Work out the finished part from the listing and answer in its coordinate system (mm). Face numbers are marked on the shaded views. Coordinates: 2 decimals unless noted, no trailing zeros. Loops run counter-clockwise (first coordinate to the right, second up) from the corner with the lowest first, then second, coordinate; pieces in that order, holes last.
Autodesk Inventor part; units mm, degrees
ref_plane "YZ Plane" through (0, 0, 0) normal (1, 0, 0) x (0, 1, 0)
ref_plane "XZ Plane" through (0, 0, 0) normal (0, 1, 0) x (-1, 0, 0)
ref_plane "XY Plane" through (0, 0, 0) normal (0, 0, 1) x (1, 0, 0)
sketch "Sketch1" plane through (0, 0, 0) normal (0, 1, 0) x (-1, 0, 0)
  circle A0 centre (0, 0) radius 18.5
  dimension "d0" = 37
extrude "Extrusion1" add sketch "Sketch1" along normal blind 55.8
sketch "Sketch2" plane through (0, 55.8, 0) normal (0, 1, 0) x (1, 0, 0)
  circle A0 centre (0, 0) radius 6
  dimension "d3" = 12
extrude "Extrusion2" add sketch "Sketch2" along normal blind 5
sketch "Sketch3" plane through (0, 60.8, 0) normal (0, 1, 0) x (1, 0, 0)
  circle A0 centre (0, 0) radius 3
  line L0 (-2.5, -3) -> (3, -3)
  line L1 (3, -3) -> (3, 3)
  line L2 (3, 3) -> (-2.5, 3)
  line L3 (-2.5, 3) -> (-2.5, -3)
  point P0 (-2.5, 1.6583)
  point P1 (-2.5, -1.6583)
  dimension "d6" = 6
  dimension "d7" = 5.5
extrude "Extrusion3" add sketch "Sketch3" along normal blind 14 contours A0 L3 picked at (0.6006, -0.3482)
sketch "Sketch4" plane through (0, 0, 0) normal (0, -1, 0) x (1, 0, 0)
  circle A0 centre (0, 0) radius 17.5
  circle A1 centre (0, 0) radius 18.5
  dimension "d27" = 1
extrude "Extrusion4" cut sketch "Sketch4" against normal blind 1 contours A0
sketch "Sketch5" plane through (0, 1, 0) normal (0, -1, 0) x (1, 0, 0)
  circle A0 centre (0, 0) radius 18.5
  circle A1 centre (0, 0) radius 5
  dimension "d13" = 10
extrude "Extrusion5" add sketch "Sketch5" along normal blind 2 contours A1
sketch "Sketch7" plane through (0, 55.8, 0) normal (0, 1, 0) x (1, 0, 0)
  line L0 (0, 25.9) -> (0, -25.9)
  point P0 (0, 0)
  point P1 (0, 15.5)
  point P2 (-13.4234, 7.75)
  point P3 (-13.4234, -7.75)
  point P4 (0, -15.5)
  point P5 (13.4234, -7.75)
  point P6 (13.4234, 7.75)
  dimension "d35" = 15.5
  dimension "d38" = 360
hole "Hole1" at (-13.4234, 55.8, -7.75) at (-13.4234, 55.8, 7.75) at (13.4234, 55.8, 7.75) at (13.4234, 55.8, -7.75) at (0, 55.8, -15.5) at (0, 55.8, 15.5) direction (0, -1, 0) diameter 2.459 depth 8.8 tip angle 118
sketch "Sketch8" plane through (0, 1, 0) normal (0, -1, 0) x (1, 0, 0)
  line L0 (-11.5, -1.5) -> (-11, -1.5)
  line L1 (-11, -1.5) -> (-11, 1.5)
  line L2 (-11, 1.5) -> (-11.5, 1.5)
  line L3 (-11.5, 1.5) -> (-11.5, -1.5)
  line L4 (11, -1.5) -> (11.5, -1.5)
  line L5 (11.5, -1.5) -> (11.5, 1.5)
  line L6 (11.5, 1.5) -> (11, 1.5)
  line L7 (11, 1.5) -> (11, -1.5)
  circle A0 centre (0, 0) radius 5
  circle A1 centre (0, 0) radius 17.5
  line L8 (0, -17.5) -> (0, 17.5) construction
  point P0 (-11, 0)
  point P1 (11, 0)
  dimension "d30" = 23
  dimension "d31" = 0.5
  dimension "d32" = 0.5
  dimension "d33" = 3
  dimension "d34" = 3
extrude "Extrusion7" add sketch "Sketch8" along normal blind 6.5 contours L3 L2 L1 L0 | L7 L6 L5 L4
properties part number "Motor24V_V1" material "Steel"
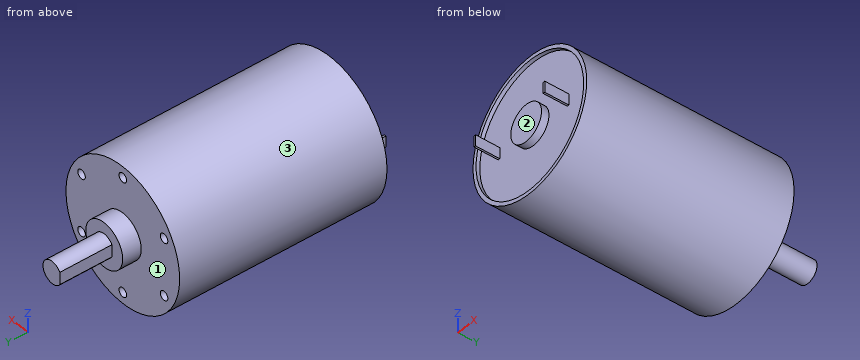
1. A cutting plane is placed at C-C, the plane y = 59.5. Give the vertices of the cut face in (x, z), then the cut area to 3 significant figures.
2. Each of these flat-tipped pins is pushed along its axis until it touches: P1, Ø0.9, axis at y = -3.5, z = 0.5, coming from the +X side; P2, Ø6, axis at x = 14, z = 3, coming from the +Y side; P3, Ø1.5, axis at y = -1, z = 0, coming from the -X side. Where does it stop, or does it pass through?
3. Determine the mould class of the marked faces 1, 2 and 3 for opening direction X: released by +X, released by -X, zero draft, split by the parting line, or undercut.
4. Straight lines are drawn through the part: probe 1 along Z at (x, y) = (0, 52); probe 2 along Z at (x, y) = (0, 0.45); probe 3 along X at (y, z) = (54, 7.75). For each, find the intervals that lie inside material, in ascending order.
5. A cutting plane is placed at B-B, the plane x = 8. Give the vertices of the cut face in (y, z).
6. A cutting plane is placed at D-D, the plane z = 13.5. Give the vertices of the cut face in (x, y), then the cut area to 3 significant figures.
7. A cutting plane is placed at A-A, the plane z = 0. Give the vertices of the cut face in (x, y).
Answers below:
1. outline: circle Ø12 at (0, 0)
1. area: 113 mm2
2. P1: stops at x = 11.5
2. P2: stops at y = 55.8
2. P3: stops at x = -11.5
3. face 1: zero draft
3. face 2: undercut
3. face 3: split by the parting line
4. probe 1: z = -18.5 to -16.73, -14.27 to 14.27, 16.73 to 18.5
4. probe 2: z = -18.5 to -17.5, -5 to 5, 17.5 to 18.5
4. probe 3: x = -16.8 to -14.65, -12.19 to 12.19, 14.65 to 16.8
5. outline: (0, -16.68) - (55.8, -16.68) - (55.8, 16.68) - (0, 16.68) - (0, 15.56) - (1, 15.56) - (1, -15.56) - (0, -15.56) - close
6. outline: (-12.65, 0) - (-11.14, 0) - (-11.14, 1) - (11.14, 1) - (11.14, 0) - (12.65, 0) - (12.65, 55.8) - (-12.65, 55.8) - close
6. area: 1,390 mm2
7. outline: (-18.5, 0) - (-17.5, 0) - (-17.5, 1) - (-11.5, 1) - (-11.5, -5.5) - (-11, -5.5) - (-11, 1) - (-5, 1) - (-5, -1) - (5, -1) - (5, 1) - (11, 1) - (11, -5.5) - (11.5, -5.5) - (11.5, 1) - (17.5, 1) - (17.5, 0) - (18.5, 0) - (18.5, 55.8) - (6, 55.8) - (6, 60.8) - (3, 60.8) - (3, 74.8) - (-2.5, 74.8) - (-2.5, 60.8) - (-6, 60.8) - (-6, 55.8) - (-18.5, 55.8) - close
